CAD build for the part. Positions are in the model's coordinates, mm. A direction names the side the tool comes from. Round coordinates to 2 decimals unless told otherwise and drop trailing zeros. Order: outer loops, then holes, each group sorted by start corner. A loop starts at its lowest first (then second) coordinate and runs counter-clockwise, first axis right, second up.
Autodesk Inventor part; units mm, degrees
sketch "Sketch1" plane through (0, 0, 0) normal (0, 0, 1) x (1, 0, 0)
  line L0 (0, 2.8582) -> (0, -2.8582) construction
  line L1 (-5.7775, 0) -> (5.7775, 0) construction
  circle A0 centre (0, 0) radius 13.75
  line L2 (5, 12.8087) -> (5, 25)
  line L3 (5, 25) -> (-5, 25)
  line L4 (-5, 25) -> (-5, 12.8087)
  line L5 (0, 32.75) -> (0, -21.5) construction
  point P0 (0, 20)
  dimension "d0" = 27.5
  dimension "d1" = 20
  dimension "d2" = 5
  dimension "d3" = 5
  dimension "d4" = 5
extrude "Extrusion1" add sketch "Sketch1" along normal blind 2.5
sketch "Sketch2" plane through (0, 0, 2.5) normal (0, 0, 1) x (1, 0, 0)
  line L0 (-5, 25) -> (-5, 12.8087)
  arc A0 (-5, 12.8087) -> (5, 12.8087) centre (0, 0) ccw
  line L1 (-5, 12.8087) -> (-5, 25)
  line L2 (-5, 25) -> (5, 25)
  line L3 (5, 25) -> (5, 12.8087)
  point P0 (0, 20)
  dimension "d7" = 5
  dimension "d8" = 5
hole "Hole1" at (0, 20, 2.5) direction (0, 0, -1) diameter 4.2 end through all
fillet "Fillet1" radius 5 2 edges at (-5, 25, 1.25) (5, 25, 1.25)
sketch "Sketch3" plane through (0, 0, 0) normal (1, 0, 0) x (0, 1, 0)
  line L0 (12.8087, 2.5) -> (-13.75, 2.5)
  line L1 (-7.5, 2.5) -> (7.5, 2.5)
  line L2 (7.5, 2.5) -> (7.5, 1)
  line L3 (7.5, 1) -> (-7.5, 1)
  line L4 (-7.5, 1) -> (-7.5, 2.5)
  line L5 (0, 3) -> (0, -0.5)
  line L6 (22.1, 2.5) -> (25, 2.5)
  line L7 (25, 2.5) -> (25, 0)
  line L8 (25, 0) -> (22.1, 0)
  line L9 (22.1, 0) -> (22.1, 2.5)
  line L10 (17.9, 0) -> (-13.75, 0)
  line L11 (-13.75, 0) -> (-13.75, 2.5)
  line L12 (-13.75, 2.5) -> (17.9, 2.5)
  line L13 (17.9, 2.5) -> (17.9, 0)
  point P0 (0, 0)
  point P1 (7.5, 2.5)
  dimension "d17" = 15
  dimension "d18" = 7.5
  dimension "d19" = 1.5
extrude "Extrusion2" cut sketch "Sketch3" along normal mid plane 7 contours L2 L3 L5 L0 | L5 L3 L4 L0
sketch "Sketch4" plane through (-3.5, 7.5, 2.5) normal (0, -1, 0) x (1, 0, 0)
  line L0 (15.0244, -2.5) -> (-8.0244, -2.5)
  line L1 (-8.0244, -2.5) -> (-8.0244, 0)
  line L2 (-8.0244, 0) -> (0, 0)
  line L3 (0, 0) -> (7, 0)
  line L4 (7, 0) -> (7, -1.5)
  line L5 (7, -1.5) -> (0, -1.5)
  line L6 (0, 0) -> (0, -1.5)
  line L7 (15.0244, 0) -> (15.0244, -2.5)
  line L8 (7, 0) -> (15.0244, 0)
  line L9 (0, 0) -> (7, -1.5)
  point P0 (3.5, -2.5)
extrude "Extrusion3" add sketch "Sketch4" along normal up to surface (15 mm away) contours L9 L5 L6
equation "\"d18\" = 0.5 * d17"
properties part number "Filler Cap" material "S235"
1. Pin check, flat tips, straight feed: P1, Ø1, axis at x = -2, y = 0.5, coming from the +Z side; P2, Ø1.5, axis at y = 15, z = 0.5, coming from the +X side; P3, Ø0.5, axis at x = 1.5, z = 2, coming from the +Y side; P4, Ø2.5, axis at x = 0, y = 20, coming from the -Z side. Stop position of each tip, or through.
2. Cut at C-C, the plane x = -9.25. Write the cut outline in (y, z), and give its area (3 significant figures).
3. Mould opens along X. For faces 4 (the face through (0, 2, 0)), 5 (the face through (-3, 24, 1)), 6 (the face through (2, 7.5, 2)), 7 (the face through (5, 16, 1)) say: released by +X, released by -X, zero draft, split by the parting line, or undercut.
4. Tool access for faces 1 (the face through (-5, 16, 1)), 2 (the face through (3.5, 0, 2)), 3 (the face through (6, 6, 2.5)): list every direction of +Z, -Z, +X, -X, +Y, -Y with a clear straight run to the whole face (end or side of a thin tool).
5. Cut at D-D, the plane y = 7. Write the cut outline in (x, z), and give its area (3 significant figures).
6. Drill centre lines: line 1 (Y direction, x = 0, z = 1.9); line 2 (X direction, y = 20, z = 1.2); line 3 (Y direction, x = 0, z = 1.4). Where is each one in solid material? Low to high.
7. Cut at A-A, the plane y = 0. Write the cut outline in (x, z), and give its area (3 significant figures).
Outcome:
1. P1: stops at z = 2.29
1. P2: stops at x = 5
1. P3: stops at y = 24.84
1. P4: passes through
2. outline: (-10.17, 0) - (10.17, 0) - (10.17, 2.5) - (-10.17, 2.5) - close
2. area: 50.9 mm2
3. face 4: zero draft
3. face 5: released by -X
3. face 6: undercut
3. face 7: released by +X
4. face 1: +Z, -Z, -X, +Y
4. face 2: +Z
4. face 3: +Z, +X, -X, +Y, -Y
5. outline: (-11.83, 0) - (11.83, 0) - (11.83, 2.5) - (3.5, 2.5) - (3.5, 1) - (-3.5, 2.5) - (-11.83, 2.5) - close
5. area: 53.9 mm2
6. line 1: y = -13.75 to -7.5, 7.5 to 17.9, 22.1 to 25
6. line 2: x = -5 to -2.1, 2.1 to 5
6. line 3: y = -13.75 to 17.9, 22.1 to 25
7. outline: (-13.75, 0) - (13.75, 0) - (13.75, 2.5) - (3.5, 2.5) - (3.5, 1) - (-3.5, 2.5) - (-13.75, 2.5) - close
7. area: 63.5 mm2
